CAD build for the part. Positions are in the model's coordinates, mm. A direction names the side the tool comes from. Coordinates: 2 decimals unless noted, no trailing zeros. Order: outer loops, then holes, each group sorted by start corner. A loop starts at its lowest first (then second) coordinate and runs counter-clockwise, first axis right, second up. Notation, with made-up numbers: M -34,-7 L -20,-7 A35 cw -20,28 Z; hole C 36,57 d3. An arc over 180 degrees is marked long. Write item = value, one per line.
from build123d import *

# Parameters (mm, degrees)
BOSS_EXTRUDE1_DEPTH = 50
SKETCH2_R           = 11.5
BOSS_EXTRUDE2_DEPTH = 150


with BuildPart() as part:
    # Sketch1 → Boss-Extrude1 (new body)
    with BuildSketch(Plane(origin=(0, 0, 0), x_dir=(1, 0, 0), z_dir=(0, 1, 0))):
        Polygon((155, -200), (155, -75), (90, -75), (90, 75), (155, 75), (155, 200), (-155, 200), (-155, -200), align=None)
    extrude(amount=BOSS_EXTRUDE1_DEPTH)

    # Sketch2 → Boss-Extrude2 (add)
    with BuildSketch(Plane.XY.offset(-75)):
        with Locations(Location((143.5, 38.5, 0), (0, 0, 90))):
            Circle(SKETCH2_R)
    extrude(amount=BOSS_EXTRUDE2_DEPTH)


solid = part.part
(1) Slice it at A-A, the plane x = 97. Write the cut outline in (y, z), then the cut area to 3 significant figures.
Evaluation:
outline = M 0,-200 L 50,-200 L 50,-75 L 0,-75 Z; M 0,75 L 50,75 L 50,200 L 0,200 Z
area = 12,500 mm²
(2) Pin check, flat tips, straight feed: pin 1 Ø8 at (y, z) = (6.5, 38) entering from +X; pin 2 Ø4 at (x, z) = (18.5, 147) entering from -Y; pin 3 Ø4 at (y, z) = (31, 4) entering from +X. Stop position of each tip, or through.
Evaluation:
pin_1 = 90
pin_2 = 0
pin_3 = 153.6
(3) Tool access for faces 4 (the face through (135.73, 30.02, -1.05)), 5 (the face through (90, 25, 1)), 6 (the face through (153, 48, -75)): list every direction of +Z, -Z, +X, -X, +Y, -Y with a clear straight run to the whole face (end or side of a thin tool).
Evaluation:
face_4 = none
face_5 = +Y, -Y
face_6 = +X, +Y
(4) Pull direction X, two halves, no side cores. Call faces 1 (the face through (-2, 0, -3)), 2 (the face through (123, 25, 75)), 3 (the face through (-155, 25, -3)): +X half, -X half, draft (parallel to the pull), parting line (faces both ways), or undercut.
Evaluation:
face_1 = draft
face_2 = undercut
face_3 = -X half
(5) Slice it at C-C, the plane z = 5. Write the cut outline in (x, y).
Evaluation:
outline = M -155,0 L 90,0 L 90,50 L -155,50 Z; C 143.5,38.5 d23
(6) Slice it at B-B, the plane y = 6. Write the cut outline in (x, z).
Evaluation:
outline = M -155,-200 L 155,-200 L 155,-75 L 90,-75 L 90,75 L 155,75 L 155,200 L -155,200 Z
(7) Wall check: line 1 (Z direction, x = 131, y = 37); line 2 (X direction, y = 4.5, z = 19.5); line 3 (X direction, y = 34.5, z = 14). Give the ranges that are in metal, low to high. Write a range as from..to.
Evaluation:
line_1 = -200..-75, 75..200
line_2 = -155..90
line_3 = -155..90, 132.72..154.28
